The drawing under review shows one solid part. Ordinate dimensions are in mm from its lowest x, y, z. A direction names the side the tool comes from. Coordinates: 2 decimals unless noted, no trailing zeros. Write each loop counter-clockwise with the first axis right and the second up, starting at its lowest first coordinate (ties: lowest second). Pieces come first, ordered by that corner, then holes.
1) For P1, Ø6, axis at y = 10.5, z = 10, coming from the -X side; P2, Ø1, axis at x = 5, z = 9.5, coming from the +Y side; P3, Ø6, axis at y = 5.5, z = 25, coming from the +X side, all flat-tipped, find the tip position at first contact; note any pin that passes through.
2) Add section A-A, the plane z = 22. State the section outline as (x, y) points.
3) Add section D-D, the plane z = 12.5. State the section outline as (x, y) points.
4) For line 1 (X direction, y = 17.5, z = 19.5), list the stretches that pass through material, from the lowest coordinate up.
5) Add section B-B, the plane x = 10.5. State the section outline as (y, z) points.
6) Machinability: for the marked faces 1 and 2, which of the approach directions +Z, -Z, +X, -X, +Y, -Y give a long, thin tool a straight path to every point of the face, cutting with its end or side? Answer none if there is none.
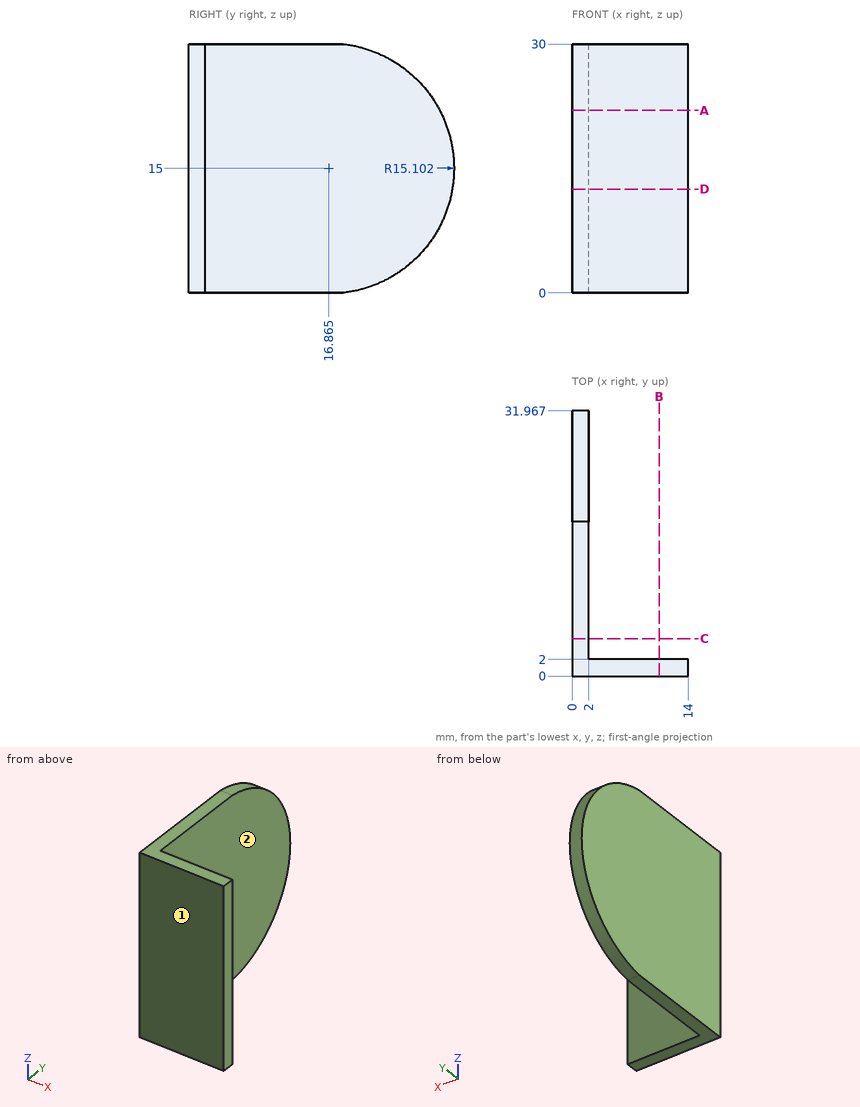
Geometry results:
1. P1: stops at x = 0
1. P2: stops at y = 2
1. P3: stops at x = 2
2. outline: (0, 0) - (14, 0) - (14, 2) - (2, 2) - (2, 30.25) - (0, 30.25) - close
3. outline: (0, 0) - (14, 0) - (14, 2) - (2, 2) - (2, 31.76) - (0, 31.76) - close
4. line 1: x = 0 to 2
5. outline: (0, 0) - (2, 0) - (2, 30) - (0, 30) - close
6. face 1: +Z, -Z, +X, -X, -Y
6. face 2: +Z, -Z, +X, +Y
